Part print with two shaded views. Sizes in mm from the minimum x, y, z corner. Round coordinates to 2 decimals unless told otherwise and drop trailing zeros. Loops run counter-clockwise (first coordinate to the right, second up) from the corner with the lowest first, then second, coordinate; pieces in that order, holes last.
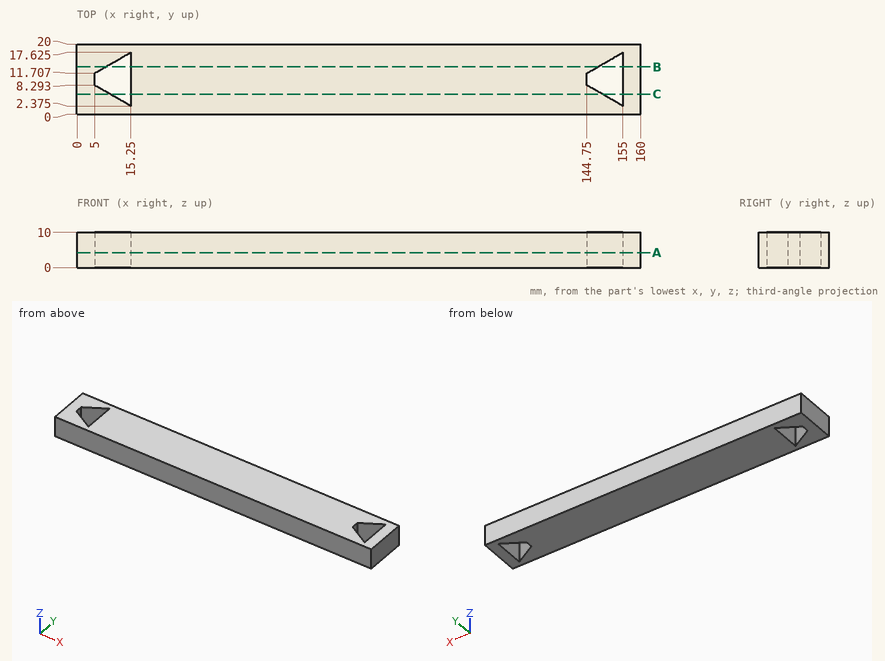
Item 1: Wall check: L1, parallel to X at y = 2.5, z = 8.75; L2, parallel to X at y = 14, z = 1.5; L3, parallel to Y at x = 7, z = 3.5. Give the ranges that are in metal, low to high.
Verdict:
L1: x = 0 to 15.03, 15.25 to 154.78, 155 to 160
L2: x = 0 to 8.97, 15.25 to 148.72, 155 to 160
L3: y = 0 to 7.14, 12.86 to 20
Item 2: Cut at C-C (y = 5.75). List the corners of the cut face in (x, z), plus the area to 3 significant figures.
Verdict:
outline: (0, 0) - (9.4, 0) - (9.4, 10) - (0, 10) - close; (15.25, 0) - (149.15, 0) - (149.15, 10) - (15.25, 10) - close; (155, 0) - (160, 0) - (160, 10) - (155, 10) - close
area: 1,480 mm2
Item 3: Cut at B-B (y = 13.5). State how many separate pieces and enclosed holes the cut face has, plus the area to 3 significant figures.
Verdict:
separate pieces: 3
enclosed holes: 0
area: 1,460 mm2
Item 4: Cut at A-A (z = 4.25). List the corners of the cut face in (x, y) (3 decimals).
Verdict:
outline: (0, 0) - (160, 0) - (160, 20) - (0, 20) - close; hole (5, 8.293) - (15.25, 2.375) - (15.25, 17.625) - (5, 11.707) - close; hole (144.75, 8.293) - (155, 2.375) - (155, 17.625) - (144.75, 11.707) - close
Item 5: Flat gauge pin, fed straight in: P1, Ø6, axis at x = 29.5, y = 5, coming from the -Z side. Where does the tip first touch, or does it go through?
Verdict:
P1: stops at z = 0
